Build history of the part. All positions in model axes, mm. A direction names the side the tool comes from. Give positions to 0.01 mm unless a question says otherwise; leave off trailing zeros. Order: outer loops, then holes, each group sorted by start corner. A loop starts at its lowest first (then second) coordinate and runs counter-clockwise, first axis right, second up. Notation, with made-up numbers: (68, 87.25) - (111, 87.25) arc R34 ccw to (111, 122.25) - close; hole circle Ø1 at (-30.75, -28). An arc over 180 degrees is marked (long way). Write each question's results on one line, items separated by ' | '. Start each with the question number.
Autodesk Inventor part; units mm, degrees
ref_plane "IP1_XY" through (0, 0, 0) normal (1, 0, 0) x (0, 0, -1)
ref_plane "IP1_YZ" through (0, 0, 0) normal (0, 0, -1) x (0, 1, 0)
ref_plane "IP1_ZX" through (0, 0, 0) normal (0, 1, 0) x (1, 0, 0)
sketch "Skizze_1" plane through (0, 0, 0) normal (0, 0, 1) x (1, 0, 0)
  line L0 (5.6, 0) -> (-0.9, 0)
  line L1 (-0.9, 0) -> (-0.9, 8.4)
  line L2 (-0.9, 8.4) -> (5.6, 8.4)
  line L3 (5.6, 8.4) -> (5.6, 0)
  line L4 (5.6, 0) -> (-0.9, 0)
revolve "Revolution1" add sketch "Skizze_1" angle 360 about axis through (5.6, 0, 0) along (1, 0, 0)
sketch "Sketch_6" plane through (0, 0, 0) normal (0, 0, 1) x (1, 0, 0)
  line L0 (5.6, 0) -> (-0.9, 0)
  line L1 (-0.9, 8.4) -> (-0.9, 5.25)
  line L2 (-0.9, 5.25) -> (-0.4, 5.25)
  line L3 (-0.4, 5.25) -> (-0.4, 8.4)
  line L4 (-0.4, 8.4) -> (-0.9, 8.4)
revolve "Revolution2" cut sketch "Sketch_6" angle 360 about axis through (5.6, 0, 0) along (1, 0, 0)
sketch "Skizze_4" plane through (0, 0, 0) normal (0, 0, 1) x (1, 0, 0)
  line L0 (5.4, 0) -> (-0.9, 0)
  line L1 (-0.9, 0) -> (-0.9, 4)
  line L2 (-0.9, 4) -> (-0.2235, 3.3235)
  line L3 (-0.2235, 3.3235) -> (4.7235, 3.3235)
  line L4 (4.7235, 3.3235) -> (5.4, 4)
  line L5 (5.4, 4) -> (5.6, 4)
  line L6 (5.6, 4) -> (5.6, 0)
  line L7 (5.6, 0) -> (-0.9, 0)
revolve "Revolution3" cut sketch "Skizze_4" angle 360 about axis through (5.4, 0, 0) along (1, 0, 0)
thread "Thread1"
sketch "Sketch_1" plane through (0, 0, 0) normal (0, 0, 1) x (1, 0, 0)
  line L0 (0, 0) -> (-0.9, 0)
  line L1 (-0.9, 8.4) -> (-0.9, 5.25)
  line L2 (-0.9, 5.25) -> (0, 5.25)
  line L3 (0, 5.25) -> (0, 8.4)
  line L4 (0, 8.4) -> (-0.9, 8.4)
revolve "Revolution4" cut sketch "Sketch_1" angle 360 about axis through (0, 0, 0) along (1, 0, 0)
sketch "Sketch_2" plane through (0, 0, 0) normal (0, 0, 1) x (1, 0, 0)
  line L0 (5.6, 0) -> (-0.9, 0)
  line L1 (-0.9, 14.69) -> (-0.9, 7)
  line L2 (-0.9, 7) -> (0, 7)
  line L3 (0, 7) -> (0.3751, 8.4)
  line L4 (0.3751, 8.4) -> (5.2249, 8.4)
  line L5 (5.2249, 8.4) -> (5.6, 7)
  line L6 (5.6, 7) -> (6.5, 7)
  line L7 (6.5, 7) -> (6.5, 14.69)
  line L8 (6.5, 14.69) -> (-0.9, 14.69)
revolve "Revolution5" cut sketch "Sketch_2" angle 360 about axis through (5.6, 0, 0) along (1, 0, 0)
sketch "Sketch_3" plane through (0, 0, 0) normal (0, 0, 1) x (1, 0, 0)
  line L0 (5.6, 0) -> (5.4, 0)
  line L1 (5.4, 0) -> (5.4, 5.25)
  line L2 (5.4, 5.25) -> (5.6, 5.25)
  line L3 (5.6, 5.25) -> (5.6, 0)
  line L4 (5.6, 0) -> (5.4, 0)
revolve "Revolution6" cut sketch "Sketch_3" angle 360 about axis through (5.6, 0, 0) along (1, 0, 0)
sketch "Skizze_3" plane through (-0.5, 0, 0) normal (1, 0, 0) x (0, 0, -1)
  line L0 (-1.7321, -7.0829) -> (0, -8.0829)
  line L1 (0, -8.0829) -> (1.7321, -7.0829)
  line L2 (1.7321, -7.0829) -> (-1.7321, -7.0829)
sketch "Skizze_9" plane through (-0.5, 0, 0) normal (1, 0, 0) x (0, 0, -1)
  line L0 (-7, 2.0415) -> (-5.2679, 5.0415)
  line L1 (-5.2679, 5.0415) -> (-7, 4.0415)
  line L2 (-7, 4.0415) -> (-7, 2.0415)
sketch "Skizze_10" plane through (-0.5, 0, 0) normal (1, 0, 0) x (0, 0, -1)
  line L0 (5.2679, 5.0415) -> (7, 2.0415)
  line L1 (7, 2.0415) -> (7, 4.0415)
  line L2 (7, 4.0415) -> (5.2679, 5.0415)
extrude "Extrusion1" add sketch "Skizze_3" along normal blind 2.1667
extrude "Extrusion2" add sketch "Skizze_9" along normal blind 2.1667
extrude "Extrusion3" add sketch "Skizze_10" along normal blind 2.1667
sketch "Skizze_7" plane through (0, 0, 0) normal (1, 0, 0) x (0, 1, 0)
  line L0 (15.38, 15.38) -> (-15.38, 15.38)
  line L1 (-15.38, 15.38) -> (-15.38, -15.38)
  line L2 (-15.38, -15.38) -> (15.38, -15.38)
  line L3 (15.38, -15.38) -> (15.38, 15.38)
  line L4 (-4.0415, 7) -> (-8.0829, 0)
  line L5 (-8.0829, 0) -> (-4.0415, -7)
  line L6 (-4.0415, -7) -> (4.0415, -7)
  line L7 (4.0415, -7) -> (8.0829, 0)
  line L8 (8.0829, 0) -> (4.0415, 7)
  line L9 (4.0415, 7) -> (-4.0415, 7)
extrude "Extrusion4" cut sketch "Skizze_7" along normal mid plane 13
ref_plane "IP1_XY" through (0, 0, 0) normal (1, 0, 0) x (0, 0, -1)
ref_plane "IP1_YZ" through (0, 0, 0) normal (0, 0, -1) x (0, 1, 0)
ref_plane "IP1_ZX" through (0, 0, 0) normal (0, 1, 0) x (1, 0, 0)
ref_plane "IP2_XY" through (5.6, 0, 0) normal (1, 0, 0) x (0, 0, -1)
ref_plane "IP2_YZ" through (5.6, 0, 0) normal (0, 0, -1) x (0, 1, 0)
ref_plane "IP2_ZX" through (5.6, 0, 0) normal (0, 1, 0) x (1, 0, 0)
properties part number "WLD-NUT DIN929 M8"
Item 1: Cut at A-A, the plane x = 1.5. List the corners of the cut face in (y, z), then the cut area to 3 significant figures.
Item 2: Which spindle directions (+Z, -Z, +X, -X, +Y, -Y) get a long thin tool onto all of the face, cutting with end or side? Do faces 1 (the flat face through (-0.5, 3.8, -6.4)), 2 (the flat face through (0, 3, 5)), 3 (the flat face through (-0.5, -7.5, 0)). Say none if no direction does.
Item 3: Two-plate mould, pull along Z, no slides. Class faces 4 (the conical face through (5.55, 7.18, 0.16)), 5 (the flat face through (-0.215, 3.521, 6.146)), 6 (the flat face through (5.4, -4, -2)), 7 (the flat face through (3, 0, -7)): +Z half, -Z half, draft (parallel to the pull), parting line (faces both ways), or undercut.
Item 4: Flat gauge pins, fed straight in: pin 1 Ø7.5 at (y, z) = (0, 0) entering from -X; pin 2 Ø2 at (x, y) = (5, -6) entering from -Z; pin 3 Ø0.5 at (y, z) = (3, 6) entering from -X. Where does each tip first touch, or does it go through?
Item 5: Probe line 1 along Z through (x, y) = (2.6, 0); line 2 along X through (y, z) = (-4.75, 4.75); line 3 along X through (y, z) = (-5, 1.5). List the from-to ranges inside material, lowest first. Write a range as from..to.
Values found:
1) outline: (-8.08, 0) - (-4.04, -7) - (4.04, -7) - (8.08, 0) - (4.04, 7) - (-4.04, 7) - close; hole circle Ø6.65 at (0, 0) | area: 135 mm2
2) face 1: -Z, -X, +Y, -Y | face 2: -X | face 3: +Z, -Z, -X, -Y
3) face 4: parting line | face 5: undercut | face 6: undercut | face 7: -Z half
4) pin 1: stops at x = -0.65 | pin 2: stops at z = -5.34 | pin 3: stops at x = 0
5) line 1: z = -7..-3.32, 3.32..7 | line 2: x = 0..5.6 | line 3: x = -0.9..5.4
